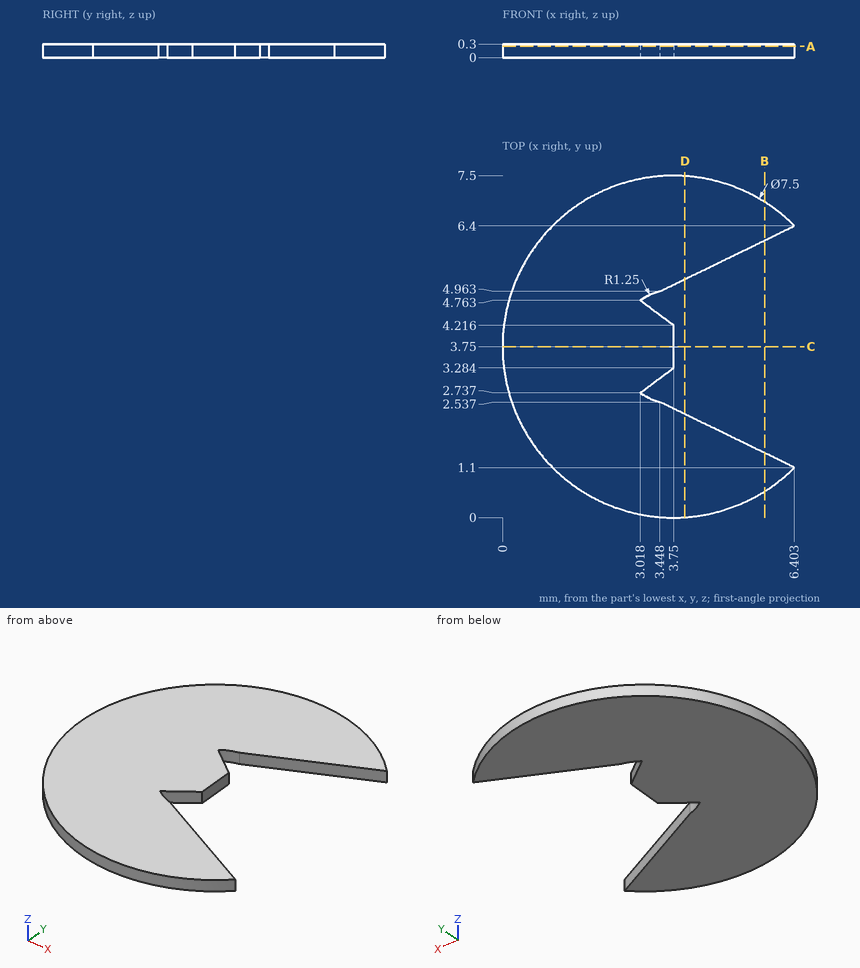
Answer from the drawing. Dimensions are ordinates in mm from the lowest x, y and z of the part. Round coordinates to 2 decimals unless told otherwise and drop trailing zeros. Loops run counter-clockwise (first coordinate to the right, second up) from the corner with the lowest first, then second, coordinate; pieces in that order, holes last.
Q1. Section C-C on y = 3.75 is taken. Write down the section's boundary in (x, z).
Q2. Section A-A on z = 0.25 is taken. Write down the section's boundary in (x, y).
Q3. Section B-B on x = 5.75 is taken. Write down the section's boundary in (y, z).
Q4. Consider probe 1 along Y at (x, z) = (3.5, 0.25) (1 decimal); probe 2 along X at (y, z) = (6.5, 0.25); probe 3 along X at (y, z) = (6, 0.2). Determine where each line is inside the solid, lowest interval first.
Q5. Section D-D on x = 4 is taken. Write down the section's boundary in (y, z).
Output:
1. outline: (0, 0) - (3.75, 0) - (3.75, 0.3) - (0, 0.3) - close
2. outline: (3.02, 2.74) - (3.75, 3.28) - (3.75, 4.22) - (3.02, 4.76) arc R1.25 cw to (3.45, 4.96) - (6.4, 6.4) arc R3.75 ccw (long way) to (6.4, 1.1) - (3.45, 2.54) arc R1.25 cw to start
3. outline: (0.58, 0) - (1.42, 0) - (1.42, 0.3) - (0.58, 0.3) - close; (6.08, 0) - (6.92, 0) - (6.92, 0.3) - (6.08, 0.3) - close
4. probe 1: y = 0 to 2.5, 3.1 to 4.4, 5 to 7.5
4. probe 2: x = 1.2 to 6.3
4. probe 3: x = 0.75 to 5.58
5. outline: (0.01, 0) - (2.27, 0) - (2.27, 0.3) - (0.01, 0.3) - close; (5.23, 0) - (7.49, 0) - (7.49, 0.3) - (5.23, 0.3) - close
